Source: CAD feature listing. Evaluate the final solid. Frame: model axes, mm. Face numbers are marked on the shaded views. A direction names the side the tool comes from. Round coordinates to 2 decimals unless told otherwise and drop trailing zeros. Order: outer loops, then holes, each group sorted by start corner. A loop starts at its lowest first (then second) coordinate and runs counter-clockwise, first axis right, second up. Notation, with made-up numbers: (60, 88.25) -> (104, 88.25) arc R18 cw to (104, 120.25) -> close; hole circle Ø5 at (10.5, -21). An arc over 180 degrees is marked (long way). One line per item, written item: value. Start each with the question number.
1) Section C-C (z = 24). Return the cut outline in (x, y), and give its area (3 significant figures).
2) Section B-B (z = 5). Return the cut outline in (x, y) (3 decimals).
3) Pin query (flat end, axial travel): P1, Ø1, axis at x = 0, z = 16, coming from the -Y side; P2, Ø5.5, axis at x = 1, y = -1, coming from the -Z side; P3, Ø1, axis at y = -2, z = 21, coming from the +X side; P4, Ø10, axis at x = 5, y = -8.5, coming from the -Z side. Return the tip coordinate at first contact, or that it passes through.
4) Ray query, L1, parallel to Z at x = -6.25, y = -4.75; L2, parallel to Y at x = 0, z = 32; L3, parallel to Z at x = -1.5, y = -3. Return the intervals inside material, ascending.
5) Reachability of the marked faces 1, 2, 3, 4 and 5 from +Z, -Z, +X, -X, +Y, -Y: full face, straight path, thin tool, end or side. Return the list, or none.
6) Section A-A (z = 35.5). Return the cut outline in (x, y).
```python
from build123d import *

# Parameters (mm, degrees)
SKETCH2_R          = 12.258164927
CUT_EXTRUDE1_DEPTH = 12
FILLET3_R          = 0.8
FILLET6_R          = 0.8
FILLET7_R          = 0.8


with BuildPart() as part:
    # Sketch1 → Revolve1 (revolve)
    with BuildSketch(Plane(origin=(0, 0, 0), x_dir=(0, 0, -1), z_dir=(1, 0, 0))):
        with BuildLine():
            Line((0, 0), (0, 2.85))
            Line((0, 2.85), (-0.655292556, 3.985))
            Line((-0.655292556, 3.985), (-7.4, 3.985))
            ThreePointArc((-7.4, 3.985), (-7.682842712, 4.102157288), (-7.8, 4.385))
            Line((-7.8, 4.385), (-7.8, 5.5))
            Line((-7.8, 5.5), (-8.8, 6.5))
            Line((-8.8, 6.5), (-17, 6.5))
            Line((-17, 6.5), (-17.414213562, 6.085786438))
            ThreePointArc((-17.414213562, 6.085786438), (-18.06306026, 5.652240935), (-18.828427125, 5.5))
            Line((-18.828427125, 5.5), (-21.2, 5.5))
            ThreePointArc((-21.2, 5.5), (-21.765685425, 5.734314575), (-22, 6.3))
            Line((-22, 6.3), (-22, 10.5))
            ThreePointArc((-22, 10.5), (-22.146446609, 10.853553391), (-22.5, 11))
            Line((-22.5, 11), (-27, 11))
            Line((-27, 11), (-27, 10.8))
            Line((-27, 10.8), (-38.624871131, 10.8))
            Line((-38.624871131, 10.8), (-39, 9.4))
            Line((-39, 9.4), (-39, 0))
            Line((-39, 0), (0, 0))
        make_face()
    revolve(axis=Axis((0, 0, 0), (0, 0, 1)))

    # Sketch2 → Cut-Extrude1 (cut)
    with BuildSketch(Plane.XY.offset(39)):
        Circle(SKETCH2_R)
        Polygon((0, -10.969655115), (9.5, -5.484827557), (9.5, 5.484827557), (0, 10.969655115), (-9.5, 5.484827557), (-9.5, -5.484827557), align=None, mode=Mode.SUBTRACT)
    extrude(amount=-CUT_EXTRUDE1_DEPTH, mode=Mode.SUBTRACT)

    # Fillet3
    fillet3_edges = [part.edges().sort_by_distance(p)[0] for p in [
        (4.75, 8.227241336, 27),
        (-4.75, -8.227241336, 27),
    ]]
    fillet(fillet3_edges, radius=FILLET3_R)

    # Fillet6
    fillet6_edges = [part.edges().sort_by_distance(p)[0] for p in [
        (4.75, -8.227241336, 27),
        (-4.75, 8.227241336, 27),
    ]]
    fillet(fillet6_edges, radius=FILLET6_R)

    # Fillet7
    fillet7_edges = [part.edges().sort_by_distance(p)[0] for p in [
        (9.5, 0, 27),
        (-9.5, 0, 27),
    ]]
    fillet(fillet7_edges, radius=FILLET7_R)


solid = part.part
```
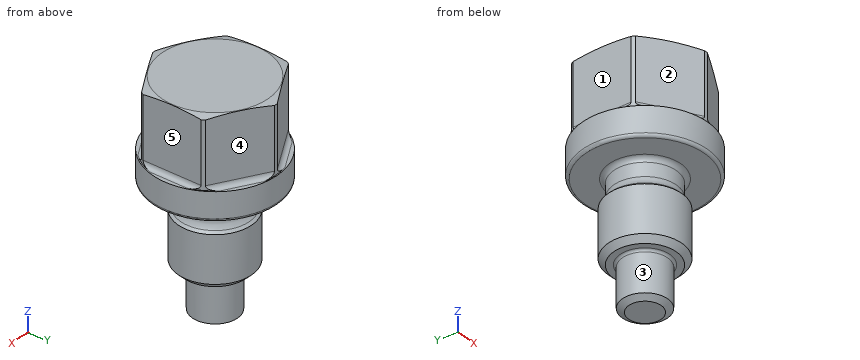
Findings:
1. outline: circle Ø22 at (0, 0)
1. area: 380 mm2
2. outline: circle Ø7.97 at (0, 0)
3. P1: y = -6.5
3. P2: z = 0
3. P3: x = 5.29
3. P4: z = 7.8
4. L1: 22 to 39
4. L2: -10.8 to 10.8
4. L3: 0.29 to 39
5. face 1: +Z, -X, +Y, -Y
5. face 2: +Z, -X, -Y
5. face 3: -Z
5. face 4: +Z, +X, +Y
5. face 5: +Z, +X, +Y, -Y
6. outline: (-9.5, -5.14) arc R10.8 ccw to (-9.2, -5.66) -> (-0.3, -10.8) arc R10.8 ccw to (0.3, -10.8) -> (9.2, -5.66) arc R10.8 ccw to (9.5, -5.14) -> (9.5, 5.14) arc R10.8 ccw to (9.2, 5.66) -> (0.3, 10.8) arc R10.8 ccw to (-0.3, 10.8) -> (-9.2, 5.66) arc R10.8 ccw to (-9.5, 5.14) -> close
